Build history of the part. All positions in model axes, mm. A direction names the side the tool comes from. Coordinates: 2 decimals unless noted, no trailing zeros. Order: outer loops, then holes, each group sorted by start corner. A loop starts at its lowest first (then second) coordinate and runs counter-clockwise, first axis right, second up. Notation, with made-up numbers: (70, 12) - (94, 12) arc R15 ccw to (94, 32) - close; hole circle Ø11 at (38, 8). An arc over 180 degrees is marked (long way). Write each question's results on one line, items separated by ' | '.
Solid Edge part; units mm, degrees
sketch "Sketch1" plane through (0, 0, 0) normal (0, -1, 0) x (1, 0, 0)
  line L0 (0, 0) -> (70, 0)
  line L1 (70, 0) -> (70, 28)
  line L2 (70, 28) -> (58, 28)
  line L3 (58, 10) -> (58, 28)
  line L4 (0, 10) -> (58, 10)
  line L5 (0, 0) -> (0, 10)
extrude "Protrusion1" add sketch "Sketch1" against normal blind 35
sketch "Sketch2" plane through (70, 17.5, 14) normal (1, 0, 0) x (0, 1, 0)
  arc A0 (-17.5, 14.1736) -> (17.5, 14) centre (0.0004, 14.1736) cw
extrude "ExtrudedProtrusion_2" add sketch "Sketch2" against normal blind 12 material side at (70, 17.587, 45.6238)
sketch "Sketch3" plane through (29, 17.5, 10) normal (0, 0, 1) x (1, 0, 0)
  line L0 (-4, 17.5) -> (-4, 5.5)
  line L1 (-4, 5.5) -> (-29, 5.5)
  line L2 (-29, 5.5) -> (-29, 17.5)
  line L3 (-29, 17.5) -> (-4, 17.5)
extrude "ExtrudedProtrusion_3" add sketch "Sketch3" along normal blind 16
sketch "Sketch4" plane through (12.5, 23, 18) normal (0, -1, 0) x (1, 0, 0)
  arc A0 (-12.5, 8) -> (12.5, 8) centre (0, 8) cw
extrude "ExtrudedProtrusion_4" add sketch "Sketch4" against normal blind 12 material side at (12.5, 23, 38.45)
sketch "Sketch5" plane through (12.5, 23, 24.25) normal (0, -1, 0) x (1, 0, 0)
  circle A0 centre (0, 1.75) radius 7.5
extrude "ExtrudedCutout_1" cut sketch "Sketch5" against normal blind 108.8355
sketch "Sketch6" plane through (70, 17.5004, 22.837) normal (1, 0, 0) x (0, 1, 0)
  circle A0 centre (0, 5.3366) radius 7.5
extrude "ExtrudedCutout_2" cut sketch "Sketch6" against normal blind 24.048
1. Two-plate mould, pull along X, no slides. Class faces 4 (the face through (0, 21, 7)), 5 (the face through (64.08, 20.96, 21.52)), 6 (the face through (29, 13, 10)): +X half, -X half, draft (parallel to the pull), parting line (faces both ways), or undercut.
Solved:
face 4: -X half | face 5: draft | face 6: undercut
2. Band-saw the part on D-D on x = 52.5. Give the cut face in (y, z), then the cut area to 3 significant figures.
Solved:
outline: (0, 0) - (35, 0) - (35, 10) - (0, 10) - close | area: 350 mm2
3. Band-saw the part on A-A on x = 12.5. Give the cut face in (y, z), then the cut area to 3 significant figures.
Solved:
outline: (0, 0) - (35, 0) - (35, 18.5) - (23, 18.5) - (23, 10) - (0, 10) - close; (23, 33.5) - (35, 33.5) - (35, 38.5) - (23, 38.5) - close | area: 512 mm2
4. Probe line 1 (X direction, y = 28, z = 26); line 2 (Z direction, x = 12.5, y = 30); line 3 (X direction, y = 23.5, z = 22.5). List the from-to ranges inside material, lowest first.
Solved:
line 1: x = 0 to 5, 20 to 25, 58 to 70 | line 2: z = 0 to 18.5, 33.5 to 38.5 | line 3: x = 0 to 5.87, 19.13 to 25, 58 to 70
5. Band-saw the part on B-B on z = 23. Give the cut face in (x, y), then the cut area to 3 significant figures.
Solved:
outline: (0, 23) - (5.63, 23) - (5.63, 35) - (0, 35) - close; (19.37, 23) - (25, 23) - (25, 35) - (19.37, 35) - close; (58, 0) - (70, 0) - (70, 12.07) - (58, 12.07) - close; (58, 22.93) - (70, 22.93) - (70, 35) - (58, 35) - close | area: 425 mm2
6. Tool access for faces 1 (the face through (25, 29, 18)), 2 (the face through (13, 23, 18)), 3 (the face through (35, 35, 7)): list every direction of +Z, -Z, +X, -X, +Y, -Y with a clear straight run to the whole face (end or side of a thin tool).
Solved:
face 1: +Z, +Y, -Y | face 2: +Z, -X, -Y | face 3: +Z, -Z, +X, -X, +Y
7. Band-saw the part on C-C on y = 29.5. Give the cut face in (x, z), then the cut area to 3 significant figures.
Solved:
outline: (0, 0) - (70, 0) - (70, 40.91) - (58, 40.91) - (58, 10) - (25, 10) - (25, 26) arc R12.5 ccw to (0, 26) - close; hole circle Ø15 at (12.5, 26) | area: 1,540 mm2
8. Drop flat-ended pins along their axis: pin 1 Ø19 at (x, z) = (33, 20) entering from +Y; pin 2 Ø24 at (x, z) = (12.5, 26) entering from -Y; pin 3 Ø3 at (x, y) = (43, 9) entering from +Z; pin 4 Ø17.5 at (x, y) = (30.5, 19) entering from +Z. Give the stop position or say it passes through.
Solved:
pin 1: stops at y = 35 | pin 2: stops at y = 23 | pin 3: stops at z = 10 | pin 4: stops at z = 33.2
